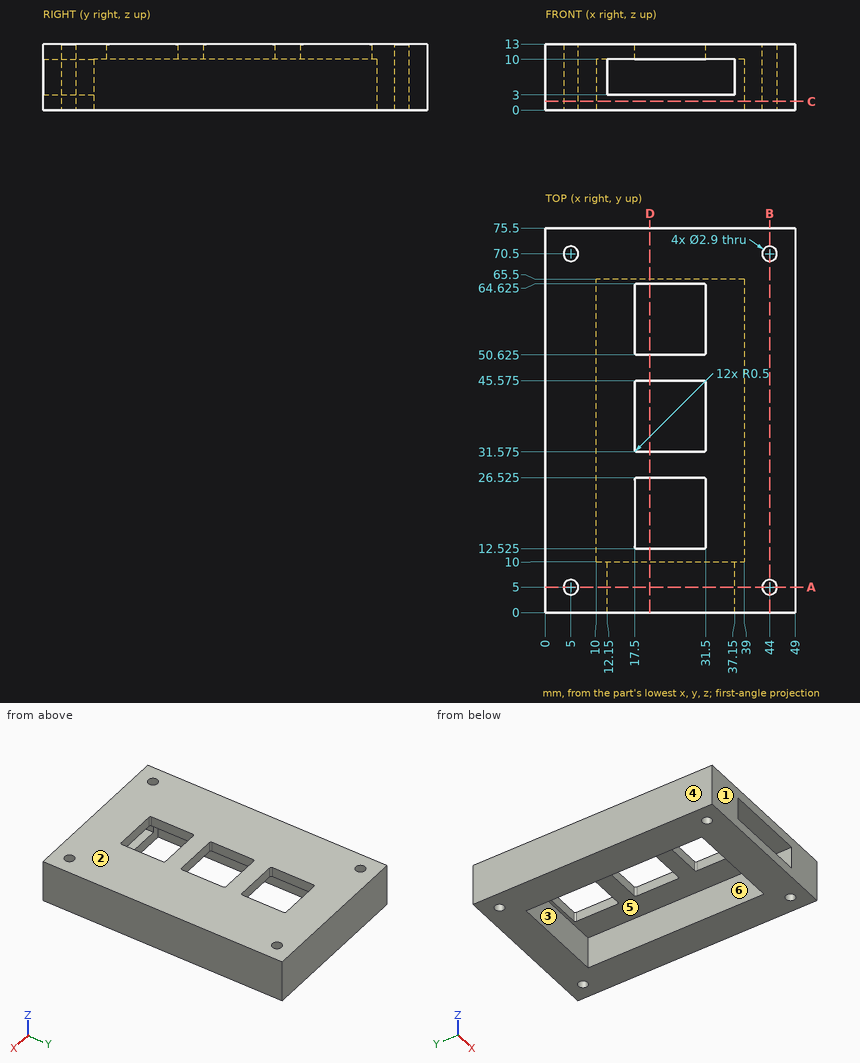
Part print with two shaded views. Sizes in mm from the minimum x, y, z corner. A direction names the side the tool comes from. Round coordinates to 2 decimals unless told otherwise and drop trailing zeros. Loops run counter-clockwise (first coordinate to the right, second up) from the corner with the lowest first, then second, coordinate; pieces in that order, holes last. Notation, with made-up numbers: (24, 38.25) - (73, 38.25) arc R19 ccw to (73, 72.25) - close; hole circle Ø11 at (62, 41.5). An arc over 180 degrees is marked (long way). Answer as a JSON object with one key per item and string values.
Item 1: Band-saw the part on B-B on x = 44. List the corners of the cut face in (y, z).
Output:
{"outline": "(0, 0) - (3.55, 0) - (3.55, 13) - (0, 13) - close; (6.45, 0) - (69.05, 0) - (69.05, 13) - (6.45, 13) - close; (71.95, 0) - (75.5, 0) - (75.5, 13) - (71.95, 13) - close"}
Item 2: Band-saw the part on A-A on y = 5. List the corners of the cut face in (x, z).
Output:
{"outline": "(0, 0) - (3.55, 0) - (3.55, 13) - (0, 13) - close; (6.45, 0) - (42.55, 0) - (42.55, 13) - (6.45, 13) - close; (45.45, 0) - (49, 0) - (49, 13) - (45.45, 13) - close; hole (12.15, 3) - (37.15, 3) - (37.15, 10) - (12.15, 10) - close"}
Item 3: Band-saw the part on D-D on x = 20.5. List the corners of the cut face in (y, z) (3 decimals).
Output:
{"outline": "(0, 0) - (10, 0) - (10, 3) - (0, 3) - close; (0, 10) - (12.525, 10) - (12.525, 13) - (0, 13) - close; (26.525, 10) - (31.575, 10) - (31.575, 13) - (26.525, 13) - close; (45.575, 10) - (50.625, 10) - (50.625, 13) - (45.575, 13) - close; (64.625, 10) - (65.5, 10) - (65.5, 0) - (75.5, 0) - (75.5, 13) - (64.625, 13) - close"}
Item 4: Pin check, flat tip, straight feed: pin 1 (2.5 mm diameter, centred on x = 5, y = 70.5, fed in from -Z). Stop position of the tip, or through.
Output:
{"pin 1": "through"}
Item 5: Tool access for the marked faces 4, 5 and 6: list every direction of +Z, -Z, +X, -X, +Y, -Y with a clear straight run to the whole face (end or side of a thin tool).
Output:
{"face 4": "+Z, -Z, -X, +Y, -Y", "face 5": "none", "face 6": "-Z"}
Item 6: Pull direction Y, two halves, no side cores. Call the marked faces 1, 2 and 3: pulls with the +Y half, pulls with the -Y half, needs draft (parallel to the pull), parting line crosses it, or undercut.
Output:
{"face 1": "pulls with the -Y half", "face 2": "needs draft", "face 3": "undercut"}
Item 7: Band-saw the part on C-C on z = 1.75. List the corners of the cut face in (x, y).
Output:
{"outline": "(0, 0) - (49, 0) - (49, 75.5) - (0, 75.5) - close; hole circle Ø2.9 at (5, 5); hole circle Ø2.9 at (5, 70.5); hole (10, 10) - (39, 10) - (39, 65.5) - (10, 65.5) - close; hole circle Ø2.9 at (44, 5); hole circle Ø2.9 at (44, 70.5)"}
Item 8: Wall check: L1, parallel to Y at x = 44, z = 9.5; L2, parallel to Y at x = 23.5, z = 12 (3 decimals); L3, parallel to X at y = 13, z = 11. Give the ranges that are in metal, low to high.
Output:
{"L1": "0 to 3.55, 6.45 to 69.05, 71.95 to 75.5", "L2": "0 to 12.525, 26.525 to 31.575, 45.575 to 50.625, 64.625 to 75.5", "L3": "0 to 17.5, 31.5 to 49"}
